For this review, use the dimensioned drawing (mm, ordinates from the lowest corner) and the shaded views. A direction names the side the tool comes from. Give positions to 0.01 mm unless a question says otherwise; leave off trailing zeros. Loops run counter-clockwise (first coordinate to the right, second up) from the corner with the lowest first, then second, coordinate; pieces in that order, holes last. Notation, with made-up numbers: M -39,49.5 L -35,49.5 A34 ccw -35,81.5 Z; hole C 2,0 d8. An arc over 180 degrees is marked long. Use one line per item in the form item = value. Start each with the question number.
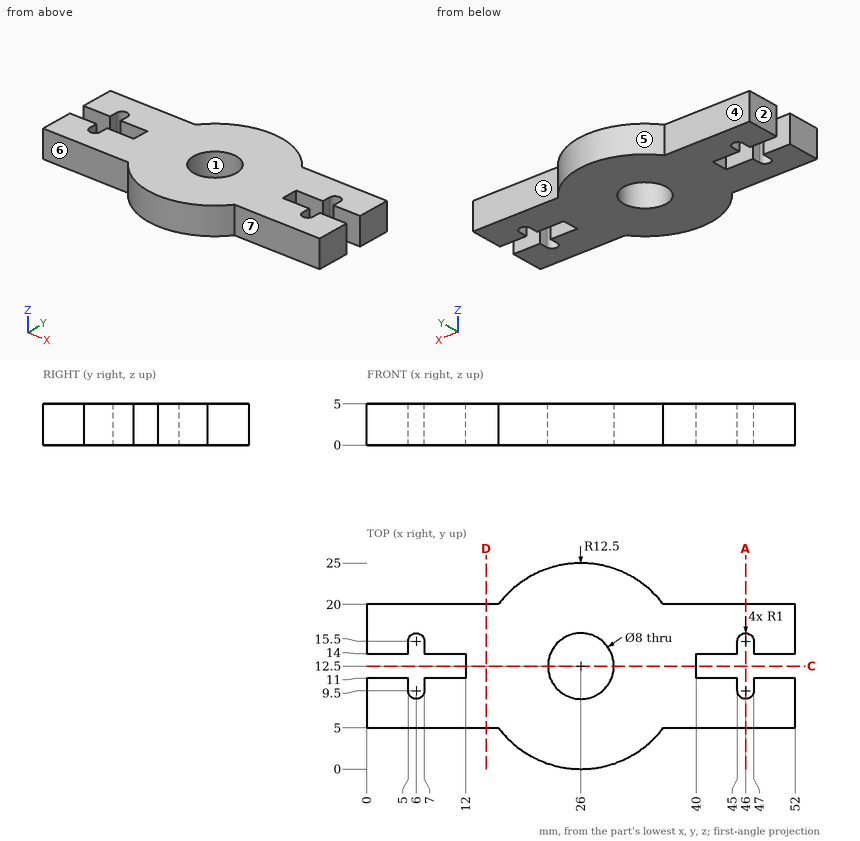
Q1. Wall thickness on probe 1 along Y at (x, z) = (26, 1.2); probe 2 along Y at (x, z) = (48, 2.4); probe 3 along X at (y, z) = (9.75, 4.6): over which ranges is each line inside the solid? List them lowest first.
Q2. Take a section at D-D on x = 14.5. Give the boundary of the cut face in (y, z).
Q3. The part is to be moulded in two halves that separate along Y. For the marked faces 1, 2 and 3, say which applies: pulls with the +Y half, pulls with the -Y half, needs draft (parallel to the pull), parting line crosses it, or undercut.
Q4. For the marked faces 4, 5, 6 and 7, list the 3-axis set-ups (+Z, -Z, +X, -X, +Y, -Y) from which the entire face can be reached by the end or side of a thin tool; tool diameter is ignored.
Q5. Take a section at A-A on x = 46. Give the boundary of the cut face in (y, z).
Q6. Clearance check with flat-ended pins moving along their axes: pin 1 Ø1.5 at (x, z) = (6, 1.5) entering from +Y; pin 2 Ø1.5 at (y, z) = (12.5, 2.5) entering from -X; pin 3 Ø2 at (x, z) = (24, 1) entering from -Y. State where each tip first meets the part, or that it passes through.
Q7. Take a section at C-C on y = 12.5. Give the boundary of the cut face in (x, z).
Response values:
q1.probe_1 = 0 to 8.5, 16.5 to 25
q1.probe_2 = 5 to 11, 14 to 20
q1.probe_3 = 0 to 5, 7 to 23.1, 28.9 to 45, 47 to 52
q2.outline = M 5,0 L 20,0 L 20,5 L 5,5 Z
q3.face_1 = undercut
q3.face_2 = needs draft
q3.face_3 = pulls with the +Y half
q4.face_4 = +Z, -Z, -X, +Y
q4.face_5 = +Z, -Z, +Y
q4.face_6 = +Z, -Z, -X, -Y
q4.face_7 = +Z, -Z, +X, -Y
q5.outline = M 5,0 L 8.5,0 L 8.5,5 L 5,5 Z; M 16.5,0 L 20,0 L 20,5 L 16.5,5 Z
q6.pin_1 = 20
q6.pin_2 = 12
q6.pin_3 = 0.04
q7.outline = M 12,0 L 22,0 L 22,5 L 12,5 Z; M 30,0 L 40,0 L 40,5 L 30,5 Z
